```python
from build123d import *

# Parameters (mm, degrees)
F0_R     = 38.1
F1_DEPTH = 12.7
F2_R     = 7.62
F3_DEPTH = 12.7
F6_DEPTH = 38.1


# Not quite as in the source:
# - a feature names something its author has since deleted; it is built from what else it names


with BuildPart() as f1:
    # F0 (on Top) → F1 (new body)
    with BuildSketch(Plane.XY):
        Circle(F0_R)
    extrude(amount=F1_DEPTH)

    # F2 (on face) → F3 (join)
    with BuildSketch(Plane.XY.offset(12.7)):
        Circle(F2_R)
    extrude(amount=F3_DEPTH)

    # F4 (on Right) → F5 (revolve)
    with BuildSketch(Plane.YZ):
        Polygon((0, 38.1), (0, 25.4), (7.62, 25.4), (3.81, 38.1), align=None)
    revolve(axis=Axis((0, 0, 31.75), (0, 0, 1)))

    # F6 (add): a face of the model
    f6_faces = [f1.faces().sort_by_distance(p)[0] for p in [
        (0, 0, 38.1),
    ]]
    extrude(f6_faces, amount=F6_DEPTH)


solid = f1.part
```
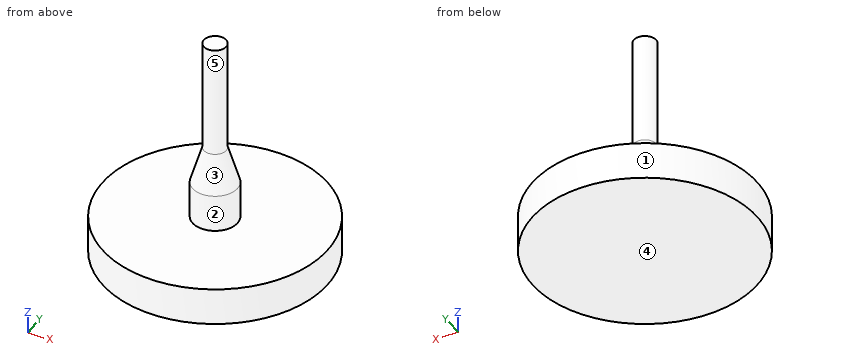
Read the model definition and answer for the solid it produces. Units are mm, in the model's axes. Face numbers are marked on the shaded views. A direction names the side the tool comes from. Coordinates: 2 decimals unless noted, no trailing zeros. Write each loop counter-clockwise with the first axis right and the second up, starting at its lowest first coordinate (ties: lowest second). Pieces come first, ordered by that corner, then holes. Notation, with made-up numbers: (69, 41) -> (81, 41) arc R21 cw to (81, 63) -> close; hole circle Ø7 at (-39.75, -30.5). An arc over 180 degrees is marked (long way). Answer as a JSON object with one key per item and string values.
Q1. The part is cut by section D-D on z = 31. Give the vertices of the cut face in (x, y).
The answers:
{"outline": "circle Ø11.88 at (0, 0)"}
Q2. Determine the mould class of the marked faces 3, 4 and 5 for opening direction Z: pulls with the +Z half, pulls with the -Z half, needs draft (parallel to the pull), parting line crosses it, or undercut.
The answers:
{"face 3": "pulls with the +Z half", "face 4": "pulls with the -Z half", "face 5": "needs draft"}
Q3. A tool of negligible diameter and unlimited length cuts with its end or side. For the marked faces 1 and 2, from which of +Z, -Z, +X, -X, +Y, -Y can it reach the whole face along a straight path? Write none if from no direction.
The answers:
{"face 1": "+Z, -Z", "face 2": "+Z"}
Q4. Consider line 1 (Z direction, x = 19, y = 23.5); line 2 (Y direction, x = 0.5, z = 10.5); line 3 (Y direction, x = -3, z = 49). Determine where each line is inside the solid, lowest interval first. Write a range as [from, to].
The answers:
{"line 1": "z = [0, 12.7]", "line 2": "y = [-38.1, 38.1]", "line 3": "y = [-2.35, 2.35]"}
Q5. The part is cut by section A-A on x = 0. Give the vertices of the cut face in (y, z).
The answers:
{"outline": "(-38.1, 0) -> (38.1, 0) -> (38.1, 12.7) -> (7.62, 12.7) -> (7.62, 25.4) -> (3.81, 38.1) -> (3.81, 76.2) -> (-3.81, 76.2) -> (-3.81, 38.1) -> (-7.62, 25.4) -> (-7.62, 12.7) -> (-38.1, 12.7) -> close"}
Q6. Flat-ended cylindrical pins translate along their axes: pin 1 Ø10 at (x, z) = (11, 28.5) entering from +Y; pin 2 Ø4 at (x, z) = (12.5, 12) entering from -Y; pin 3 Ø8 at (x, z) = (-5, 32.5) entering from +Y; pin 4 Ø3 at (x, y) = (-21, 12) entering from -Z. Find the tip coordinate at first contact, or state that the pin passes through.
The answers:
{"pin 1": "stops at y = 3.49", "pin 2": "stops at y = -36.62", "pin 3": "stops at y = 5.96", "pin 4": "stops at z = 0"}
Q7. The part is cut by section C-C on z = 60.5. Give the vertices of the cut face in (x, y), then the cut area to 3 significant figures.
The answers:
{"outline": "circle Ø7.62 at (0, 0)", "area": "45.6 mm2"}
